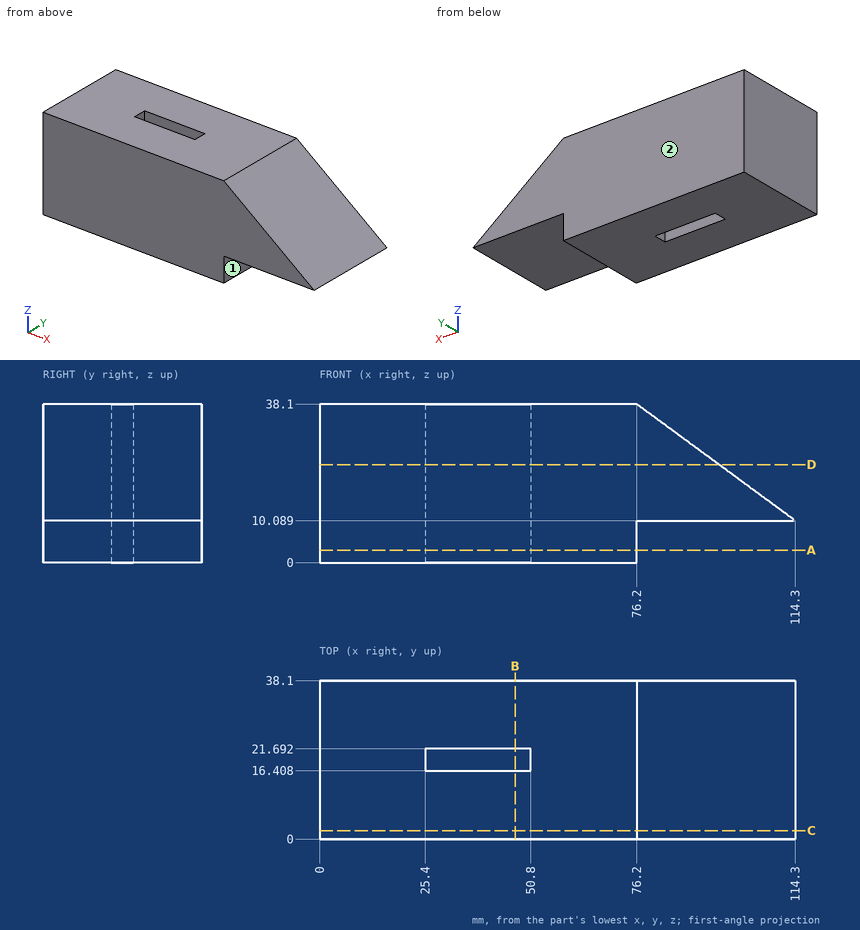
Here's the drawing with two shaded views (mm, measured from the low corner). I have some questions. A direction names the side the tool comes from. Coordinates: 2 decimals unless noted, no trailing zeros. Loops run counter-clockwise (first coordinate to the right, second up) from the corner with the lowest first, then second, coordinate; pieces in that order, holes last. Notation, with made-up numbers: (-30, -10.5) - (-9, -10.5) arc R30 ccw to (-9, 26.5) - close; hole circle Ø4 at (-24, -30). An arc over 180 degrees is marked (long way). Answer as CSV lines item,"result". Start each with the question number.
1) Which directions (+Z, -Z, +X, -X, +Y, -Y) give clear straight access to the entire face, cutting with the end or side of a thin tool? Please do the marked faces 1 and 2.
2) Suppose I cut it at C-C (y = 2). Please give me the cut outline in (x, z), plus the area to 3 significant figures.
3) I need wall thicknesses on line 1 (Y direction, x = 30, z = 24); line 2 (X direction, y = 9, z = 9.5); line 3 (X direction, y = 19, z = 29) (1 decimal). Which ranges of each line are inside material? Lowest first, please. Write a range as from..to.
4) Suppose I cut it at B-B (x = 47). Please give me the cut outline in (y, z), plus the area to 3 significant figures.
5) For pin 1 (10 mm diameter, centred on x = 103, y = 6.5, fed in from -Z); pin 2 (2.5 mm diameter, centred on y = 18, z = 26.5, fed in from +X); pin 3 (3 mm diameter, centred on y = 21, z = 3, fed in from +X), each with a flat end and sliding along its axis, tell me the tip position at first contact or that it passes through.
6) Suppose I cut it at A-A (z = 3). Please give me the cut outline in (x, y).
7) Suppose I cut it at D-D (z = 23.5). Please give me the cut outline in (x, y), plus the area to 3 significant figures.
Check result:
1,face 1,"-Z, +X, +Y, -Y"
1,face 2,"+Z, -Z, +X, -X, +Y"
2,outline,"(0, 0) - (76.2, 0) - (76.2, 10.09) - (114.3, 10.09) - (76.2, 38.1) - (0, 38.1) - close"
2,area,"3,440 mm²"
3,line 1,"y = 0..16.41, 21.69..38.1"
3,line 2,"x = 0..76.2"
3,line 3,"x = 0..25.4, 50.8..88.6"
4,outline,"(0, 0) - (16.41, 0) - (16.41, 38.1) - (0, 38.1) - close; (21.69, 0) - (38.1, 0) - (38.1, 38.1) - (21.69, 38.1) - close"
4,area,"1,250 mm²"
5,pin 1,"stops at z = 10.09"
5,pin 2,"stops at x = 93.68"
5,pin 3,"stops at x = 76.2"
6,outline,"(0, 0) - (76.2, 0) - (76.2, 38.1) - (0, 38.1) - close; hole (25.4, 16.41) - (50.8, 16.41) - (50.8, 21.69) - (25.4, 21.69) - close"
7,outline,"(0, 0) - (96.06, 0) - (96.06, 38.1) - (0, 38.1) - close; hole (25.4, 16.41) - (50.8, 16.41) - (50.8, 21.69) - (25.4, 21.69) - close"
7,area,"3,530 mm²"
